Work out the finished part from the listing and answer in its coordinate system (mm). Coordinates: 2 decimals unless noted, no trailing zeros. Loops run counter-clockwise (first coordinate to the right, second up) from the corner with the lowest first, then second, coordinate; pieces in that order, holes last. Notation, with made-up numbers: (60.25, -40) - (119.25, -40) arc R10 ccw to (119.25, -32) - close; hole circle Ø3 at (-21, 68). An arc over 180 degrees is marked (long way). Write each question's results on one line, items separated by ' | '. Start each with the question number.
Item 1: Section B-B, the plane z = 4.5 is taken. Write down the section's boundary in (x, y), plus the area to 3 significant figures.
Item 2: For a pull along Y with two mould halves and no side action, classify faces 1 (the face through (0.5, -9.99, -15.65)), 2 (the face through (0.493, -0.202, -17.537)), 3 (the face through (1, -6, 0)) as +Y half, -Y half, draft (parallel to the pull), parting line (faces both ways), or undercut.
Item 3: Consider probe 1 along Z at (x, y) = (0.3, 0); probe 2 along Y at (x, z) = (0.8, 6); probe 3 along Z at (x, y) = (0.45, 3.5). Determine where each line is inside the solid, lowest interval first. Write a range as [from, to].
Item 4: Section A-A, the plane y = 0 is taken. Write down the section's boundary in (x, z), plus the area to 3 significant figures.
Autodesk Inventor part; units mm, degrees
ref_plane "YZ Plane" through (0, 0, 0) normal (1, 0, 0) x (0, 1, 0)
ref_plane "XZ Plane" through (0, 0, 0) normal (0, 1, 0) x (-1, 0, 0)
ref_plane "XY Plane" through (0, 0, 0) normal (0, 0, 1) x (1, 0, 0)
sketch "Sketch1" plane through (0, 0, 0) normal (1, 0, 0) x (0, 1, 0)
  circle A0 centre (0, 0) radius 5.5
  line L0 (3, 18.5) -> (-3, 18.5)
  line L1 (-13, 8.5) -> (-13, -8.5)
  line L2 (-3, -18.5) -> (3, -18.5)
  line L3 (13, -8.5) -> (13, 8.5)
  line L4 (13, 18.5) -> (-13, -18.5) construction
  line L5 (-13, 18.5) -> (13, -18.5) construction
  circle A1 centre (0, 16) radius 1.55
  line L6 (0, 0) -> (10.4906, 0) construction
  circle A2 centre (0, -16) radius 1.55
  line L7 (0, 0) -> (0, 32) construction
  arc A3 (13, 8.5) -> (3, 18.5) centre (3, 8.5) ccw
  arc A4 (-3, 18.5) -> (-13, 8.5) centre (-3, 8.5) ccw
  arc A5 (-13, -8.5) -> (-3, -18.5) centre (-3, -8.5) ccw
  arc A6 (3, -18.5) -> (13, -8.5) centre (3, -8.5) ccw
  dimension "d0" = 11
  dimension "d1" = 2.5
  dimension "d2" = 37
  dimension "d3" = 26
  dimension "d4" = 3.1
  dimension "d5" = 10
extrude "Extrusion1" add sketch "Sketch1" along normal blind 1
fillet "Fillet1" radius 0.25 16 edges at (1, 0, 18.5) (1, -10.0711, 15.5711) (1, -13, 0) (1, -10.0711, -15.5711) (1, 0, -18.5) (1, 10.0711, -15.5711) (1, 13, 0) (1, 10.0711, 15.5711) (0, 0, 18.5) (0, -10.0711, 15.5711) (0, -13, 0) (0, -10.0711, -15.5711) (0, 0, -18.5) (0, 10.0711, -15.5711) (0, 13, 0) (0, 10.0711, 15.5711)
properties part number "Component 7 (Cover Plate)"
Answer key:
1) outline: (0, -12.75) arc R0.25 ccw to (0.25, -13) - (0.75, -13) arc R0.25 ccw to (1, -12.75) - (1, -3.16) - (0, -3.16) - close; (0, 3.16) - (1, 3.16) - (1, 12.75) arc R0.25 ccw to (0.75, 13) - (0.25, 13) arc R0.25 ccw to (0, 12.75) - close | area: 19.6 mm^2
2) face 1: -Y half | face 2: undercut | face 3: draft
3) probe 1: z = [-18.5, -17.55], [-14.45, -5.5], [5.5, 14.45], [17.55, 18.5] | probe 2: y = [-12.99, 12.99] | probe 3: z = [-18.49, -4.24], [4.24, 18.49]
4) outline: (0, -18.25) arc R0.25 ccw to (0.25, -18.5) - (0.75, -18.5) arc R0.25 ccw to (1, -18.25) - (1, -17.55) - (0, -17.55) - close; (0, -14.45) - (1, -14.45) - (1, -5.5) - (0, -5.5) - close; (0, 5.5) - (1, 5.5) - (1, 14.45) - (0, 14.45) - close; (0, 17.55) - (1, 17.55) - (1, 18.25) arc R0.25 ccw to (0.75, 18.5) - (0.25, 18.5) arc R0.25 ccw to (0, 18.25) - close | area: 19.7 mm^2
